```python
from build123d import *

# Parameters (mm, degrees)
EXTRUDE_1_DEPTH = 10


with BuildPart() as part:
    # 草图1 → 凸台-拉伸1 (new body)
    with BuildSketch(Plane.XY):
        Polygon((-51, 0), (-143.5, -410), (-36, -410), (143.5, -410), (51, 0), align=None)
        with BuildLine():
            ThreePointArc((-31.189754148, -393.74573768), (-28.949930235, -402.058616091), (-36, -407))
            ThreePointArc((-36, -407), (-43.006292692, -402.176165673), (-41, -393.909830056))
            Line((-41, -393.909830056), (-41, -387))
            ThreePointArc((-41, -387), (-35.859408171, -382.001976997), (-31.007906425, -387.281072477))
            Line((-31.007906425, -387.281072477), (-31.189754148, -393.74573768))
        make_face(mode=Mode.SUBTRACT)
        with BuildLine():
            Line((-41, -228.909830056), (-41, -222))
            ThreePointArc((-41, -222), (-36, -217), (-31, -222))
            Line((-31, -222), (-31, -228.909830056))
            ThreePointArc((-31, -228.909830056), (-36, -242), (-41, -228.909830056))
        make_face(mode=Mode.SUBTRACT)
        with BuildLine():
            Line((-41, -63.909830056), (-41, -57))
            ThreePointArc((-41, -57), (-36, -52), (-31, -57))
            Line((-31, -57), (-31, -63.909830056))
            ThreePointArc((-31, -63.909830056), (-36, -77), (-41, -63.909830056))
        make_face(mode=Mode.SUBTRACT)
        with BuildLine():
            Line((41, -57), (41, -63.909830056))
            ThreePointArc((41, -63.909830056), (36, -77), (31, -63.909830056))
            Line((31, -63.909830056), (31, -57))
            ThreePointArc((31, -57), (36, -52), (41, -57))
        make_face(mode=Mode.SUBTRACT)
        with BuildLine():
            Line((41, -387), (41, -393.909830056))
            ThreePointArc((41, -393.909830056), (35.874567803, -406.998951044), (31.189754148, -393.74573768))
            Line((31.189754148, -393.74573768), (31.007906425, -387.281072477))
            ThreePointArc((31.007906425, -387.281072477), (35.859408171, -382.001976997), (41, -387))
        make_face(mode=Mode.SUBTRACT)
        with BuildLine():
            Line((31, -228.909830056), (31, -222))
            ThreePointArc((31, -222), (36, -217), (41, -222))
            Line((41, -222), (41, -228.909830056))
            ThreePointArc((41, -228.909830056), (36, -242), (31, -228.909830056))
        make_face(mode=Mode.SUBTRACT)
    extrude(amount=EXTRUDE_1_DEPTH)


solid = part.part
```
The model under review builds one solid part; all positions refer to its coordinate system, in mm. A direction names the side the tool comes from. Round coordinates to 2 decimals unless told otherwise and drop trailing zeros. Order: outer loops, then holes, each group sorted by start corner. A loop starts at its lowest first (then second) coordinate and runs counter-clockwise, first axis right, second up. Notation, with made-up numbers: (42, 85) -> (58, 85) arc R26 ccw to (58, 117) -> close; hole circle Ø4 at (25.25, 86). An arc over 180 degrees is marked (long way). One line per item, written item: value. Start each with the question number.
Q1. Take a section at A-A (z = 6.5). Write out the cut boundary in (x, y).
Q2. Mouldability with a two-part tool opening along Y and no side actions: class faces 3 (the face through (-2, -248, 10)), 4 (the face through (-96.603, -202.13, 4.93)), 5 (the face through (-36, -77, 5)), 6 (the face through (36, -242, 5)) as released by +Y, released by -Y, zero draft, split by the parting line, or undercut.
Q3. Take a section at B-B (x = 36). Write out the cut boundary in (y, z), and give its area (3 significant figures).
Q4. Clearance check with flat-ended pins moving along their axes: pin 1 Ø2 at (y, z) = (-60.5, 3) entering from +X (3 decimals); pin 2 Ø3.5 at (y, z) = (-224, 7) entering from -X; pin 3 Ø3.5 at (y, z) = (-224, 3.5) entering from +X; pin 4 Ø19.5 at (x, y) = (36, -234.5) entering from +Z. State where each tip first meets the part, or that it passes through.
Q5. Wall thickness on line 1 (Y direction, x = 36, z = 7.5); line 2 (X direction, y = -69.5, z = 5); line 3 (X direction, y = -234.5, z = 4.75): over which ranges is each line inside the solid? List them lowest first.
Q6. Machinability: for faces 1 (the face through (1, 0, 5)), 2 (the face through (-36, -382, 5)), which of the approach directions +Z, -Z, +X, -X, +Y, -Y give a long, thin tool a straight path to every point of the face, cutting with its end or side? Answer none if there is none.
Q7. Take a section at D-D (y = -234.5). Write out the cut boundary in (x, z).
Q8. Take a section at C-C (y = -399.5). Write out the cut boundary in (x, z).
Reported:
1. outline: (-143.5, -410) -> (143.5, -410) -> (51, 0) -> (-51, 0) -> close; hole (-41, -393.91) arc R7.5 ccw (long way) to (-31.19, -393.75) -> (-31.01, -387.28) arc R5 ccw (long way) to (-41, -387) -> close; hole (-41, -228.91) arc R7.5 ccw (long way) to (-31, -228.91) -> (-31, -222) arc R5 ccw to (-41, -222) -> close; hole (-41, -63.91) arc R7.5 ccw (long way) to (-31, -63.91) -> (-31, -57) arc R5 ccw to (-41, -57) -> close; hole (31, -228.91) arc R7.5 ccw (long way) to (41, -228.91) -> (41, -222) arc R5 ccw to (31, -222) -> close; hole (31, -63.91) arc R7.5 ccw (long way) to (41, -63.91) -> (41, -57) arc R5 ccw to (31, -57) -> close; hole (31.01, -387.28) -> (31.19, -393.75) arc R7.5 ccw (long way) to (41, -393.91) -> (41, -387) arc R5 ccw (long way) to start
2. face 3: zero draft
2. face 4: released by +Y
2. face 5: undercut
2. face 6: undercut
3. outline: (-410, 0) -> (-407, 0) -> (-407, 10) -> (-410, 10) -> close; (-382, 0) -> (-242, 0) -> (-242, 10) -> (-382, 10) -> close; (-217, 0) -> (-77, 0) -> (-77, 10) -> (-217, 10) -> close; (-52, 0) -> (0, 0) -> (0, 10) -> (-52, 10) -> close
3. area: 3,350 mm2
4. pin 1: stops at x = 64.875
4. pin 2: stops at x = -101.93
4. pin 3: stops at x = 101.93
4. pin 4: stops at z = 10
5. line 1: y = -410 to -407, -382 to -242, -217 to -77, -52 to 0
5. line 2: x = -66.68 to -43.5, -28.5 to 28.5, 43.5 to 66.68
5. line 3: x = -103.91 to -43.5, -28.5 to 28.5, 43.5 to 103.91
6. face 1: +Z, -Z, +X, -X, +Y
6. face 2: +Z, -Z
7. outline: (-103.91, 0) -> (-43.5, 0) -> (-43.5, 10) -> (-103.91, 10) -> close; (-28.5, 0) -> (28.5, 0) -> (28.5, 10) -> (-28.5, 10) -> close; (43.5, 0) -> (103.91, 0) -> (103.91, 10) -> (43.5, 10) -> close
8. outline: (-141.13, 0) -> (-43.5, 0) -> (-43.5, 10) -> (-141.13, 10) -> close; (-28.5, 0) -> (28.5, 0) -> (28.5, 10) -> (-28.5, 10) -> close; (43.5, 0) -> (141.13, 0) -> (141.13, 10) -> (43.5, 10) -> close
